Work out the finished part from the listing and answer in its coordinate system (mm). Face numbers are marked on the shaded views. A direction names the side the tool comes from. Round coordinates to 2 decimals unless told otherwise and drop trailing zeros. Order: outer loops, then holes, each group sorted by start corner. A loop starts at its lowest first (then second) coordinate and runs counter-clockwise, first axis right, second up. Notation, with made-up numbers: (-24, -37.5) - (10, -37.5) arc R24 ccw to (10, -25.5) - close; hole circle Ø8 at (88, 11). An arc over 180 degrees is marked (long way). Put each result on its own line as item: value.
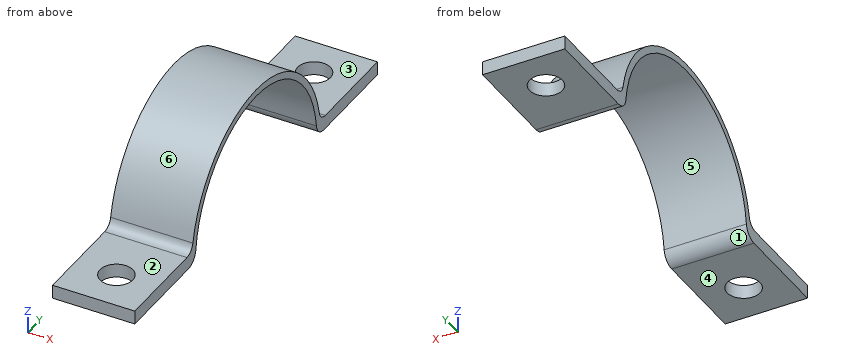
```python
from build123d import *

# Parameters (mm, degrees)
F1_DEPTH = 30
F2_R     = 4
F3_R     = 5
F4_R     = 6
F5_DEPTH = 25


with BuildPart() as f1:
    # F0 (on Right) → F1 (new body)
    with BuildSketch(Plane.YZ):
        with BuildLine():
            Line((80, 5), (42.204858, 5))
            ThreePointArc((42.204858, 5), (0, 42.5), (-42.204858, 5))
            Line((-42.204858, 5), (-80, 5))
            Line((-80, 5), (-80, 0))
            Line((-80, 0), (-40, 0))
            ThreePointArc((-40, 0), (0, 40), (40, 0))
            Line((40, 0), (80, 0))
            Line((80, 0), (80, 5))
        make_face()
    extrude(amount=F1_DEPTH)

    # F2
    f2_edges = [f1.edges().sort_by_distance(p)[0] for p in [
        (15, -42.204858, 5),
        (15, 42.204858, 5),
    ]]
    fillet(f2_edges, radius=F2_R)

    # F3
    f3_edges = [f1.edges().sort_by_distance(p)[0] for p in [
        (15, -40, 0),
        (15, 40, 0),
    ]]
    fillet(f3_edges, radius=F3_R)

    # F4 (on face) → F5 (cut)
    with BuildSketch(Plane.XY.offset(5)):
        with Locations((15, -65)):
            Circle(F4_R)
        with Locations((15.160678, 65)):
            Circle(F4_R)
    extrude(amount=-F5_DEPTH, mode=Mode.SUBTRACT)


solid = f1.part
```
1) A cutting plane is placed at C-C on x = 15. Write down the section's boundary in (y, z), then the cut area to 3 significant figures.
Findings below:
outline: (-80, 0) - (-71, 0) - (-71, 5) - (-80, 5) - close; (-59, 0) - (-44.72, 0) arc R5 ccw to (-39.75, 4.44) arc R40 cw to (39.75, 4.44) arc R5 ccw to (44.72, 0) - (59, 0) - (59, 5) - (45.62, 5) arc R4 cw to (41.7, 8.23) arc R42.5 ccw to (-41.7, 8.23) arc R4 cw to (-45.62, 5) - (-59, 5) - close; (71, 0) - (80, 0) - (80, 5) - (71, 5) - close
area: 576 mm2
2) For a pull along Y with two mould halves and no side action, classify the marked faces 4, 5 and 6 as pulls with the +Y half, pulls with the -Y half, needs draft (parallel to the pull), parting line crosses it, or undercut.
Findings below:
face 4: needs draft
face 5: undercut
face 6: parting line crosses it
3) For the marked faces 1, 2 and 3, determine the directions among +Z, -Z, +X, -X, +Y, -Y from which every point of the face is accessible in a straight line to the end or side of a thin tool.
Findings below:
face 1: -Z, +X, -X
face 2: +Z, +X, -X, -Y
face 3: +Z, +X, -X, +Y
4) A cutting plane is placed at B-B on z = 18. Write down the section's boundary in (x, y).
Findings below:
outline: (0, -38.5) - (30, -38.5) - (30, -35.72) - (0, -35.72) - close; (0, 35.72) - (30, 35.72) - (30, 38.5) - (0, 38.5) - close
5) Straight lines are drawn through the part: L1, parallel to Y at x = 15, z = 3.05; L2, parallel to Y at x = 15, z = 3.3; L3, parallel to Y at x = 17.25, z = 25. For each, find the intervals that lie inside material, in ascending order. Write a range as from..to.
Findings below:
L1: y = -80..-71, -59..-40.12, 40.12..59, 71..80
L2: y = -80..-71, -59..-40.02, 40.02..59, 71..80
L3: y = -34.37..-31.22, 31.22..34.37
6) Given pin 1 Ø15 at (x, y) = (12, 66.5) entering from +Z; pin 2 Ø1 at (x, z) = (6.5, 21) entering from +Y; pin 3 Ø4 at (x, y) = (24, -38) entering from +Z, each flat-ended and moving along its own axis, determine where each tip first touches the part or whether it passes through.
Findings below:
pin 1: stops at z = 5
pin 2: stops at y = 37.23
pin 3: stops at z = 22.59
7) A cutting plane is placed at D-D on x = 6.75. Write down the section's boundary in (y, z), then the cut area to 3 significant figures.
Findings below:
outline: (-80, 0) - (-44.72, 0) arc R5 ccw to (-39.75, 4.44) arc R40 cw to (39.75, 4.44) arc R5 ccw to (44.72, 0) - (80, 0) - (80, 5) - (45.62, 5) arc R4 cw to (41.7, 8.23) arc R42.5 ccw to (-41.7, 8.23) arc R4 cw to (-45.62, 5) - (-80, 5) - close
area: 696 mm2
8) A cutting plane is placed at A-A on y = 65. Write down the section's boundary in (x, z), then the cut area to 3 significant figures.
Findings below:
outline: (0, 0) - (9.16, 0) - (9.16, 5) - (0, 5) - close; (21.16, 0) - (30, 0) - (30, 5) - (21.16, 5) - close
area: 90.0 mm2
